Check sheet for the modelled part. Datum: model origin and axes. Units: mm. Face numbers are marked on the shaded views. Round coordinates to 2 decimals unless told otherwise and drop trailing zeros. Order: outer loops, then holes, each group sorted by start corner. A loop starts at its lowest first (then second) coordinate and runs counter-clockwise, first axis right, second up.
Q1. Mould release check, pull along Z, two halves, no side actions. Record for the marked faces 1, 2 and 3: +Z half, -Z half, draft (parallel to the pull), parting line (faces both ways), or undercut.
Q2. Cross-section at A-A on z = 1.3. Record the cut outline in (x, y), then the cut area to 3 significant figures.
Q3. Scan lines: probe 1 along Z at (x, y) = (0.3, 5.9); probe 2 along Y at (x, z) = (1.35, 1.95); probe 3 along Z at (x, y) = (-1, 6.3). Record each from-to range of solid material in increasing order.
Q4. Depth check by flat-ended pin: P1, Ø1, axis at y = 6.5, z = 1.5, coming from the -X side; P2, Ø2, axis at x = 1.5, y = 6, coming from the +Z side. Enter the tip coordinate at first touch or a pass-through.
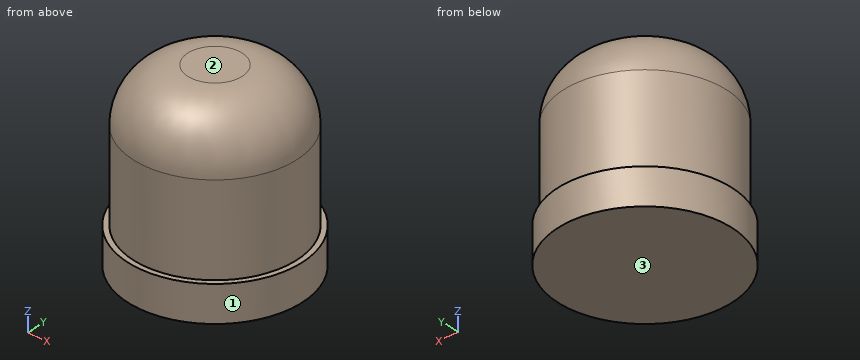
from build123d import *

# Parameters (mm, degrees)
SKETCH_1_R      = 2.25
EXTRUDE_1_DEPTH = 4
SKETCH_2_R      = 2.4
EXTRUDE_2_DEPTH = 1
FILLET_8_R      = 1.5


with BuildPart() as part:
    # Эскиз1 → Бобышка-Вытянуть1 (new body)
    with BuildSketch(Plane.XY):
        with Locations((0, 4.957015904)):
            Circle(SKETCH_1_R)
    extrude(amount=EXTRUDE_1_DEPTH)

    # Эскиз2 → Бобышка-Вытянуть2 (add)
    with BuildSketch(Plane(origin=(0, 0, 0), x_dir=(-1, 0, 0), z_dir=(0, 0, -1))):
        with Locations((0, 4.957015904)):
            Circle(SKETCH_2_R)
    extrude(amount=EXTRUDE_2_DEPTH)

    # Скругление8
    fillet_8_edges = [part.edges().sort_by_distance(p)[0] for p in [
        (-2.25, 4.957015904, 4),
    ]]
    fillet(fillet_8_edges, radius=FILLET_8_R)


solid = part.part
Results found:
1. face 1: draft
1. face 2: +Z half
1. face 3: -Z half
2. outline: circle Ø4.5 at (0, 4.96)
2. area: 15.9 mm2
3. probe 1: z = -1 to 3.98
3. probe 2: y = 3.16 to 6.76
3. probe 3: z = -1 to 3.68
4. P1: stops at x = -1.99
4. P2: stops at z = 4
